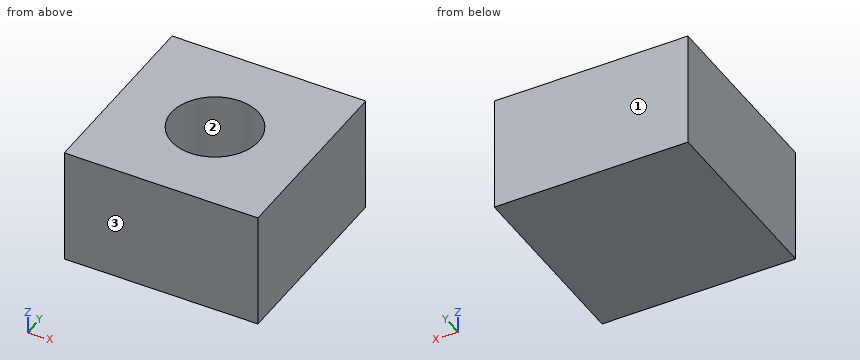
from build123d import *

# Parameters (mm, degrees)
SKETCH1_W           = 20
SKETCH1_H           = 20
SKETCH1_R           = 4.5
BOSS_EXTRUDE1_DEPTH = 10
SKETCH2_W           = 20
SKETCH2_H           = 20
BOSS_EXTRUDE2_DEPTH = 2


with BuildPart() as part:
    # Sketch1 → Boss-Extrude1 (new body)
    with BuildSketch(Plane.XY):
        Rectangle(SKETCH1_W, SKETCH1_H)
        Circle(SKETCH1_R, mode=Mode.SUBTRACT)
    extrude(amount=BOSS_EXTRUDE1_DEPTH)

    # Sketch2 → Boss-Extrude2 (add)
    with BuildSketch(Plane.XY):
        Rectangle(SKETCH2_W, SKETCH2_H)
    extrude(amount=-BOSS_EXTRUDE2_DEPTH)


solid = part.part
Geometry check sheet. Reference: the model listing, model coordinates, mm. Face numbers are marked on the shaded views. Coordinates: 2 decimals unless noted, no trailing zeros. Order: outer loops, then holes, each group sorted by start corner. A loop starts at its lowest first (then second) coordinate and runs counter-clockwise, first axis right, second up. Notation, with made-up numbers: (32, 55) - (60, 55) arc R16 ccw to (60, 77) - close; hole circle Ø8 at (56, 75.5). An arc over 180 degrees is marked (long way). One line per item, written item: value.
(1) Sectioned sample at A-A (z = 5.75). Enter the section's corners in (x, y), and give its area (3 significant figures).
Data:
outline: (-10, -10) - (10, -10) - (10, 10) - (-10, 10) - close; hole circle Ø9 at (0, 0)
area: 336 mm^2
(2) Release check for a two-part mould opening along Y. For the marked faces 1, 2 and 3 record: +Y half, -Y half, draft (parallel to the pull), parting line (faces both ways), or undercut.
Data:
face 1: +Y half
face 2: undercut
face 3: -Y half
(3) Sectioned sample at B-B (y = 0). Enter the section's corners in (x, z).
Data:
outline: (-10, -2) - (10, -2) - (10, 10) - (4.5, 10) - (4.5, 0) - (-4.5, 0) - (-4.5, 10) - (-10, 10) - close
(4) Thickness scan on probe 1 along Y at (x, z) = (0, 5.75); probe 2 along Z at (x, y) = (-3, -0.75); probe 3 along X at (y, z) = (-4, 5). Record the ranges inside material, lowest first. Write a range as from..to.
Data:
probe 1: y = -10..-4.5, 4.5..10
probe 2: z = -2..0
probe 3: x = -10..-2.06, 2.06..10
(5) Depth check by flat-ended pin: pin 1 Ø4.5 at (x, y) = (0, -1) entering from +Z. Enter the tip coordinate at first touch or a pass-through.
Data:
pin 1: stops at z = 0
